Here's how the part is built. I have some questions about the finished solid (model axes, mm). Face numbers are marked on the shaded views. A direction names the side the tool comes from. Round coordinates to 2 decimals unless told otherwise and drop trailing zeros. Write each loop counter-clockwise with the first axis right and the second up, starting at its lowest first coordinate (ties: lowest second). Pieces come first, ordered by that corner, then holes. Notation, with made-up numbers: (-0.5, 36.25) -> (19.5, 36.25) arc R17 cw to (19.5, 64.25) -> close; hole circle Ø1 at (-31.75, 65.25). An arc over 180 degrees is marked (long way). Answer as CSV lines item,"result".
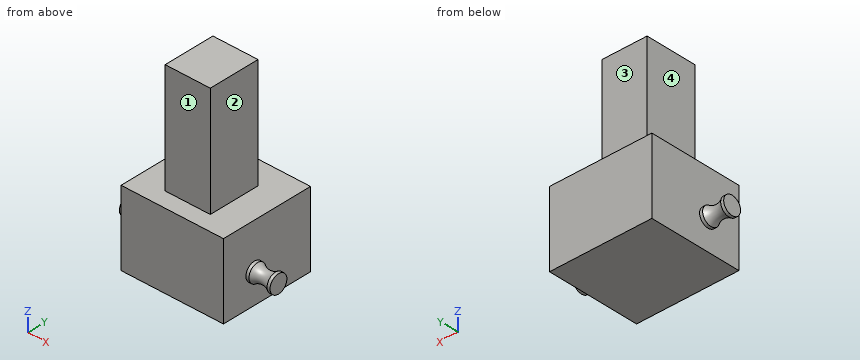
```python
from build123d import *

# Parameters (mm, degrees)
SKETCH016_W       = 17
SKETCH016_H       = 31
PAD011_DEPTH      = 15
PAD011_DEPTH_BACK = 10
SKETCH017_W       = 7.5
SKETCH017_H       = 17
PAD012_DEPTH      = 37


with BuildPart() as part:
    # Sketch014 → Revolution002 (revolve)
    with BuildSketch(Plane.XZ):
        with BuildLine():
            Line((-24, 3), (-25, 3))
            Line((-25, 3), (-25, 0))
            Line((-25, 0), (-17, 0))
            Line((-17, 0), (-17, 3))
            Line((-17, 3), (-18, 3))
            ThreePointArc((-24, 3), (-21, 2), (-18, 3))
        make_face()
    revolve(axis=Axis((0, 0, 0), (1, 0, 0)))

    # Sketch016 → Pad011 (new body, two sides)
    with BuildSketch(Plane.XY) as pad011_sk:
        with Locations((-8.5, 4.5)):
            Rectangle(SKETCH016_W, SKETCH016_H)
    extrude(amount=PAD011_DEPTH)
    extrude(pad011_sk.sketch, amount=-PAD011_DEPTH_BACK)

    # Sketch017 (on Face8 of Pad011) → Pad012 (join)
    with BuildSketch(Plane(origin=(0, 0, 15), x_dir=(-1, 0, 0), z_dir=(0, 0, 1))):
        with Locations((3.75, -3)):
            Rectangle(SKETCH017_W, SKETCH017_H)
    extrude(amount=PAD012_DEPTH)

    # Mirrored002: part across YZ


with BuildPart() as part_1:
    add(part.part)
    add(part.part.mirror(Plane.YZ))


solid = part_1.part
```
1. Suppose I cut it at A-A on x = -6. Please give me the cut outline in (y, z).
Numbers:
outline,"(-11, -10) -> (20, -10) -> (20, 15) -> (11.5, 15) -> (11.5, 52) -> (-5.5, 52) -> (-5.5, 15) -> (-11, 15) -> close"
2. Suppose I cut it at D-D on y = 8. Please give me the cut outline in (x, z).
Numbers:
outline,"(-17, -10) -> (17, -10) -> (17, 15) -> (7.5, 15) -> (7.5, 52) -> (-7.5, 52) -> (-7.5, 15) -> (-17, 15) -> close"
3. On a 3-axis mill with a long thin cutter (end or side, diameter ignored), from which of +Z, -Z, +X, -X, +Y, -Y can I reach the whole of each face in a straight line? I mean the marked faces 1, 2, 3 and 4. Say none if no direction works.
Numbers:
face 1,"+Z, +X, -X, -Y"
face 2,"+Z, +X, +Y, -Y"
face 3,"+Z, +X, -X, +Y"
face 4,"+Z, -X, +Y, -Y"
4. Suppose I cut it at B-B on z = 0. Please give me the cut outline in (x, y).
Numbers:
outline,"(-25, -3) -> (-24, -3) arc R5 cw to (-18, -3) -> (-17, -3) -> (-17, -11) -> (17, -11) -> (17, -3) -> (18, -3) arc R5 cw to (24, -3) -> (25, -3) -> (25, 3) -> (24, 3) arc R5 cw to (18, 3) -> (17, 3) -> (17, 20) -> (-17, 20) -> (-17, 3) -> (-18, 3) arc R5 cw to (-24, 3) -> (-25, 3) -> close"
5. For pin 1 Ø8 at (y, z) = (-6, 19.5) entering from -X; pin 2 Ø4.5 at (x, z) = (-1.5, 26) entering from -Y; pin 3 Ø12.5 at (y, z) = (5, 8) entering from +X, each with a flat end and sliding along its axis, tell me the tip position at first contact or that it passes through.
Numbers:
pin 1,"stops at x = -7.5"
pin 2,"stops at y = -5.5"
pin 3,"stops at x = 17"
6. If I drill on line 1 (Z direction, x = 15.5, y = 3.5); line 2 (X direction, y = 7, z = 9.5); line 3 (X direction, y = -4.5, z = 43), over which ranges is the centre line in solid material (lowest first)?
Numbers:
line 1,"z = -10 to 15"
line 2,"x = -17 to 17"
line 3,"x = -7.5 to 7.5"
7. Suppose I cut it at C-C on y = 0. Please give me the cut outline in (x, z), and give its area (3 significant figures).
Numbers:
outline,"(-25, -3) -> (-24, -3) arc R5 cw to (-18, -3) -> (-17, -3) -> (-17, -10) -> (17, -10) -> (17, -3) -> (18, -3) arc R5 cw to (24, -3) -> (25, -3) -> (25, 3) -> (24, 3) arc R5 cw to (18, 3) -> (17, 3) -> (17, 15) -> (7.5, 15) -> (7.5, 52) -> (-7.5, 52) -> (-7.5, 15) -> (-17, 15) -> (-17, 3) -> (-18, 3) arc R5 cw to (-24, 3) -> (-25, 3) -> close"
area,"1,480 mm^2"
